The listing builds one solid part. Answer for the finished solid, in the listing's coordinates (mm). Face numbers are marked on the shaded views. A direction names the side the tool comes from. Coordinates: 2 decimals unless noted, no trailing zeros. Order: outer loops, then holes, each group sorted by start corner. A loop starts at its lowest first (then second) coordinate and runs counter-clockwise, first axis right, second up. Notation, with made-up numbers: (68.25, 83) -> (115.25, 83) arc R31 cw to (115.25, 111) -> close; hole circle Ø11 at (-1, 82). An arc over 180 degrees is marked (long way). Return JSON: item names as keys, results as strings.
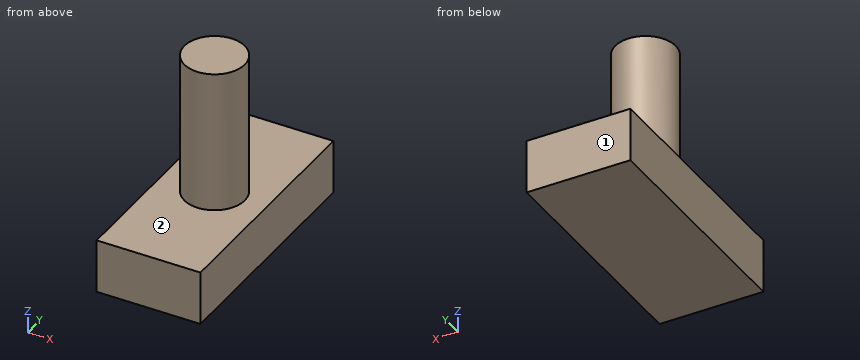
```python
from build123d import *

# Parameters (mm, degrees)
F0_W     = 111.05685
F0_H     = 57.694792
F1_DEPTH = 254
F2_R     = 32.336648
F3_DEPTH = 152.4


with BuildPart() as f1:
    # F0 (on Front) → F1 (new body)
    with BuildSketch(Plane.XZ):
        Rectangle(F0_W, F0_H)
    extrude(amount=F1_DEPTH)

    # F2 (on face) → F3 (join)
    with BuildSketch(Plane.XY.offset(28.847396)):
        with Locations((0, -127.830639)):
            Circle(F2_R)
    extrude(amount=F3_DEPTH)


solid = f1.part
```
Item 1: Flat-ended cylindrical pins translate along their axes: pin 1 (10 mm diameter, centred on x = -26.5, z = 156.5, fed in from -Y); pin 2 (4 mm diameter, centred on x = -11.5, z = 104, fed in from -Y); pin 3 (6 mm diameter, centred on x = 3, z = 74, fed in from -Y). Find the tip coordinate at first contact, or state that the pin passes through.
Answer list:
{"pin 1": "y = -151.98", "pin 2": "y = -158.74", "pin 3": "y = -160.17"}
Item 2: The part is cut by section A-A on x = 0. Determine the outline of the cut face in (y, z), plus the area to 3 significant figures.
Answer list:
{"outline": "(-254, -28.85) -> (0, -28.85) -> (0, 28.85) -> (-95.49, 28.85) -> (-95.49, 181.25) -> (-160.17, 181.25) -> (-160.17, 28.85) -> (-254, 28.85) -> close", "area": "24,500 mm2"}
Item 3: Find the intervals of material crossed by probe 1 along Z at (x, y) = (42.5, -234); probe 2 along Y at (x, z) = (1, 101); probe 3 along Y at (x, z) = (-21, 73), in increasing order.
Answer list:
{"probe 1": "-28.85 to 28.85", "probe 2": "-160.15 to -95.51", "probe 3": "-152.42 to -103.24"}
Item 4: The part is cut by section D-D on z = 159. Determine the outline of the cut face in (x, y).
Answer list:
{"outline": "circle Ø64.67 at (0, -127.83)"}
Item 5: The part is cut by section C-C on y = -227. Determine the outline of the cut face in (x, z), plus the area to 3 significant figures.
Answer list:
{"outline": "(-55.53, -28.85) -> (55.53, -28.85) -> (55.53, 28.85) -> (-55.53, 28.85) -> close", "area": "6,410 mm2"}
Item 6: Which of the six approach directions +Z, -Z, +X, -X, +Y, -Y give full straight-line access (tool end or side, diameter ignored) to the marked faces 1 and 2?
Answer list:
{"face 1": "+Z, -Z, +X, -X, +Y", "face 2": "+Z"}
Item 7: The part is cut by section B-B on y = -138.5. Determine the outline of the cut face in (x, z), plus the area to 3 significant figures.
Answer list:
{"outline": "(-55.53, -28.85) -> (55.53, -28.85) -> (55.53, 28.85) -> (30.53, 28.85) -> (30.53, 181.25) -> (-30.53, 181.25) -> (-30.53, 28.85) -> (-55.53, 28.85) -> close", "area": "15,700 mm2"}
